Input: part model. Units: mm. Frame: model coordinates. Coordinates: 2 decimals unless noted, no trailing zeros. Loops run counter-clockwise (first coordinate to the right, second up) from the corner with the lowest first, then second, coordinate; pieces in that order, holes last.
(1) Line query: L1, parallel to X at y = -34.5, z = 32. Output: solid intervals per line, ascending.
(2) Contact query for flat-ended pins moving along their axis: P1, Ø4, axis at x = -63.69, y = -62.91, coming from the +Z side; P2, Ø4, axis at x = 2.5, y = 10.5, coming from the +Z side. Output: stop coordinate, or through.
(3) Section B-B, the plane x = 33. Return loops of the section in (y, z), then the cut area to 3 significant figures.
(4) Section A-A, the plane x = 100.5. Return loops of the section in (y, z).
```python
from build123d import *

# Parameters (mm, degrees)
F0_W     = 317.5
F0_H     = 177.8
F1_DEPTH = 63.5
F2_R     = 3.302
F3_DEPTH = 31.75
F4_R     = 6.477
F5_DEPTH = 12.7


with BuildPart() as f1:
    # F0 (on Top) → F1 (new body)
    with BuildSketch(Plane.XY):
        with Locations((23.460558, -30.150112)):
            Rectangle(F0_W, F0_H)
    extrude(amount=F1_DEPTH)

    # F2 (on face) → F3 (cut)
    with BuildSketch(Plane.XY.offset(63.5)):
        with Locations((-114.488609, 38.688812)):
            Circle(F2_R)
        with Locations((-114.488609, 13.288812)):
            Circle(F2_R)
        with Locations((-114.488609, -12.111188)):
            Circle(F2_R)
        with Locations((-114.488609, -37.511188)):
            Circle(F2_R)
        with Locations((-114.488609, -62.911188)):
            Circle(F2_R)
        with Locations((-114.488609, -88.311188)):
            Circle(F2_R)
        with Locations((-89.088609, 38.688812)):
            Circle(F2_R)
        with Locations((-89.088609, 13.288812)):
            Circle(F2_R)
        with Locations((-89.088609, -12.111188)):
            Circle(F2_R)
        with Locations((-89.088609, -37.511188)):
            Circle(F2_R)
        with Locations((-89.088609, -62.911188)):
            Circle(F2_R)
        with Locations((-89.088609, -88.311188)):
            Circle(F2_R)
        with Locations((-63.688609, 38.688812)):
            Circle(F2_R)
        with Locations((-63.688609, 13.288812)):
            Circle(F2_R)
        with Locations((-63.688609, -12.111188)):
            Circle(F2_R)
        with Locations((-63.688609, -37.511188)):
            Circle(F2_R)
        with Locations((-63.688609, -62.911188)):
            Circle(F2_R)
        with Locations((-63.688609, -88.311188)):
            Circle(F2_R)
        with Locations((-38.288609, 38.688812)):
            Circle(F2_R)
        with Locations((-38.288609, 13.288812)):
            Circle(F2_R)
        with Locations((-38.288609, -12.111188)):
            Circle(F2_R)
        with Locations((-38.288609, -37.511188)):
            Circle(F2_R)
        with Locations((-38.288609, -62.911188)):
            Circle(F2_R)
        with Locations((-38.288609, -88.311188)):
            Circle(F2_R)
    extrude(amount=-F3_DEPTH, mode=Mode.SUBTRACT)

    # F4 (on face) → F5 (cut)
    with BuildSketch(Plane.XY.offset(63.5)):
        with Locations((2.748668, 38.253274)):
            Circle(F4_R)
        with Locations((2.748668, 12.853274)):
            Circle(F4_R)
        with Locations((2.748668, -12.546726)):
            Circle(F4_R)
        with Locations((2.748668, -37.946726)):
            Circle(F4_R)
        with Locations((2.748668, -63.346726)):
            Circle(F4_R)
        with Locations((2.748668, -88.746726)):
            Circle(F4_R)
        with Locations((34.498668, 38.253274)):
            Circle(F4_R)
        with Locations((34.498668, 12.853274)):
            Circle(F4_R)
        with Locations((34.498668, -12.546726)):
            Circle(F4_R)
        with Locations((34.498668, -37.946726)):
            Circle(F4_R)
        with Locations((34.498668, -63.346726)):
            Circle(F4_R)
        with Locations((34.498668, -88.746726)):
            Circle(F4_R)
        with Locations((66.248668, 38.253274)):
            Circle(F4_R)
        with Locations((66.248668, 12.853274)):
            Circle(F4_R)
        with Locations((66.248668, -12.546726)):
            Circle(F4_R)
        with Locations((66.248668, -37.946726)):
            Circle(F4_R)
        with Locations((66.248668, -63.346726)):
            Circle(F4_R)
        with Locations((66.248668, -88.746726)):
            Circle(F4_R)
        with Locations((97.998668, 38.253274)):
            Circle(F4_R)
        with Locations((97.998668, 12.853274)):
            Circle(F4_R)
        with Locations((97.998668, -12.546726)):
            Circle(F4_R)
        with Locations((97.998668, -37.946726)):
            Circle(F4_R)
        with Locations((97.998668, -63.346726)):
            Circle(F4_R)
        with Locations((97.998668, -88.746726)):
            Circle(F4_R)
        with Locations((129.748668, 38.253274)):
            Circle(F4_R)
        with Locations((129.748668, 12.853274)):
            Circle(F4_R)
        with Locations((129.748668, -12.546726)):
            Circle(F4_R)
        with Locations((129.748668, -37.946726)):
            Circle(F4_R)
        with Locations((129.748668, -63.346726)):
            Circle(F4_R)
        with Locations((129.748668, -88.746726)):
            Circle(F4_R)
        with Locations((161.498668, 38.253274)):
            Circle(F4_R)
        with Locations((161.498668, 12.853274)):
            Circle(F4_R)
        with Locations((161.498668, -12.546726)):
            Circle(F4_R)
        with Locations((161.498668, -37.946726)):
            Circle(F4_R)
        with Locations((161.498668, -63.346726)):
            Circle(F4_R)
        with Locations((161.498668, -88.746726)):
            Circle(F4_R)
    extrude(amount=-F5_DEPTH, mode=Mode.SUBTRACT)


solid = f1.part
```
Report:
1. L1: x = -135.29 to -115.84, -113.13 to -90.44, -87.73 to -65.04, -62.33 to -39.64, -36.93 to 182.21
2. P1: stops at z = 31.75
2. P2: stops at z = 50.8
3. outline: (-119.05, 0) - (58.75, 0) - (58.75, 63.5) - (44.55, 63.5) - (44.55, 50.8) - (31.95, 50.8) - (31.95, 63.5) - (19.15, 63.5) - (19.15, 50.8) - (6.55, 50.8) - (6.55, 63.5) - (-6.25, 63.5) - (-6.25, 50.8) - (-18.85, 50.8) - (-18.85, 63.5) - (-31.65, 63.5) - (-31.65, 50.8) - (-44.25, 50.8) - (-44.25, 63.5) - (-57.05, 63.5) - (-57.05, 50.8) - (-69.65, 50.8) - (-69.65, 63.5) - (-82.45, 63.5) - (-82.45, 50.8) - (-95.05, 50.8) - (-95.05, 63.5) - (-119.05, 63.5) - close
3. area: 10,300 mm2
4. outline: (-119.05, 0) - (58.75, 0) - (58.75, 63.5) - (44.23, 63.5) - (44.23, 50.8) - (32.28, 50.8) - (32.28, 63.5) - (18.83, 63.5) - (18.83, 50.8) - (6.88, 50.8) - (6.88, 63.5) - (-6.57, 63.5) - (-6.57, 50.8) - (-18.52, 50.8) - (-18.52, 63.5) - (-31.97, 63.5) - (-31.97, 50.8) - (-43.92, 50.8) - (-43.92, 63.5) - (-57.37, 63.5) - (-57.37, 50.8) - (-69.32, 50.8) - (-69.32, 63.5) - (-82.77, 63.5) - (-82.77, 50.8) - (-94.72, 50.8) - (-94.72, 63.5) - (-119.05, 63.5) - close
